Check sheet for the modelled part. Datum: model origin and axes. Units: mm. Round coordinates to 2 decimals unless told otherwise and drop trailing zeros. Order: outer loops, then holes, each group sorted by start corner. A loop starts at its lowest first (then second) coordinate and runs counter-clockwise, first axis right, second up.
```python
from build123d import *

# Parameters (mm, degrees)
F0_R     = 4.5
F0_R_2   = 30.25
F0_W     = 44
F0_H     = 3
F1_DEPTH = 4
F2_R     = 15
F3_R     = 1


with BuildPart() as f1:
    # F0 (on Top) → F1 (new body)
    with BuildSketch(Plane.XY):
        with BuildLine():
            ThreePointArc((-43.501786, 35.001786), (-35.001786, 26.501786), (-26.501786, 35.001786))
            ThreePointArc((-26.501786, 35.001786), (-28.991378, 41.012193), (-35.001786, 43.501786))
            ThreePointArc((-35.001786, 43.501786), (-39.901995, 41.94714), (-43.009713, 37.851891))
            ThreePointArc((-43.009713, 37.851891), (-43.377864, 36.447921), (-43.501786, 35.001786))
        make_face()
        with Locations((-35.001786, 35.001786)):
            Circle(F0_R, mode=Mode.SUBTRACT)
        with BuildLine():
            ThreePointArc((-35.001786, 43.501786), (-28.991378, 41.012193), (-26.501786, 35.001786))
            ThreePointArc((-26.501786, 35.001786), (-35.001786, 26.501786), (-43.501786, 35.001786))
            Line((-43.501786, 35.001786), (-43.501786, -35.001786))
            ThreePointArc((-43.501786, -35.001786), (-35.001786, -26.501786), (-26.501786, -35.001786))
            ThreePointArc((-26.501786, -35.001786), (-28.991378, -41.012193), (-35.001786, -43.501786))
            Line((-35.001786, -43.501786), (35.001786, -43.501786))
            ThreePointArc((35.001786, -43.501786), (28.991378, -28.991378), (43.501786, -35.001786))
            Line((43.501786, -35.001786), (43.501786, 35.001786))
            ThreePointArc((43.501786, 35.001786), (28.991378, 28.991378), (35.001786, 43.501786))
            Line((35.001786, 43.501786), (-35.001786, 43.501786))
        make_face()
        Circle(F0_R_2, mode=Mode.SUBTRACT)
        with BuildLine():
            Line((-43.501786, -35.001786), (-43.501786, 35.001786))
            ThreePointArc((-43.501786, 35.001786), (-43.377864, 36.447921), (-43.009713, 37.851891))
            Line((-43.009713, 37.851891), (-51.498214, 14.001786))
            Line((-51.498214, 14.001786), (-51.498214, -6.998214))
            Line((-51.498214, -6.998214), (-43.198922, -37.250552))
            ThreePointArc((-43.198922, -37.250552), (-43.42573, -36.13632), (-43.501786, -35.001786))
        make_face()
        with BuildLine():
            ThreePointArc((43.501786, 35.001786), (41.012193, 41.012193), (35.001786, 43.501786))
            ThreePointArc((35.001786, 43.501786), (28.991378, 28.991378), (43.501786, 35.001786))
        make_face()
        with Locations((35.001786, 35.001786)):
            Circle(F0_R, mode=Mode.SUBTRACT)
        with BuildLine():
            ThreePointArc((-26.501786, -35.001786), (-35.001786, -26.501786), (-43.501786, -35.001786))
            ThreePointArc((-43.501786, -35.001786), (-43.42573, -36.13632), (-43.198922, -37.250552))
            ThreePointArc((-43.198922, -37.250552), (-40.156176, -41.760651), (-35.001786, -43.501786))
            ThreePointArc((-35.001786, -43.501786), (-28.991378, -41.012193), (-26.501786, -35.001786))
        make_face()
        with Locations((-35.001786, -35.001786)):
            Circle(F0_R, mode=Mode.SUBTRACT)
        with BuildLine():
            ThreePointArc((35.001786, -43.501786), (41.012193, -41.012193), (43.501786, -35.001786))
            ThreePointArc((43.501786, -35.001786), (28.991378, -28.991378), (35.001786, -43.501786))
        make_face()
        with Locations((35.001786, -35.001786)):
            Circle(F0_R, mode=Mode.SUBTRACT)
        Polygon((35.001786, -43.501786), (-35.001786, -43.501786), (-35.001786, -45.501786), (-21.498214, -45.501786), (22.501786, -45.501786), (35.001786, -45.501786), align=None)
        with Locations((0.501786, -47.001786)):
            Rectangle(F0_W, F0_H)
    extrude(amount=F1_DEPTH)

    # F2
    f2_edges = [f1.edges().sort_by_distance(p)[0] for p in [
        (-51.498214, 14.001786, 2),
        (-51.498214, -6.998214, 2),
    ]]
    fillet(f2_edges, radius=F2_R)

    # F3
    f3_edges = [f1.edges().sort_by_distance(p)[0] for p in [
        (-35.001786, -43.501786, 2),
        (-21.498214, -45.501786, 2),
        (22.501786, -45.501786, 2),
        (35.001786, -43.501786, 2),
        (-35.001786, -45.501786, 2),
        (-21.498214, -48.501786, 2),
        (22.501786, -48.501786, 2),
        (35.001786, -45.501786, 2),
    ]]
    fillet(f3_edges, radius=F3_R)


solid = f1.part
```
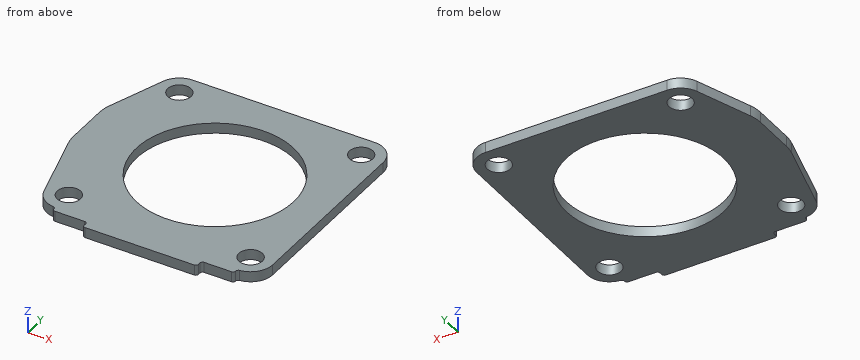
Item 1: Sectioned sample at B-B (x = 0). Record the cut outline in (y, z).
Answer:
outline: (-48.5, 0) - (-30.25, 0) - (-30.25, 4) - (-48.5, 4) - close; (30.25, 0) - (43.5, 0) - (43.5, 4) - (30.25, 4) - close
Item 2: Sectioned sample at A-A (y = 0). Record the cut outline in (x, z), and give its area (3 significant figures).
Answer:
outline: (-51.5, 0) - (-30.25, 0) - (-30.25, 4) - (-51.5, 4) - close; (30.25, 0) - (43.5, 0) - (43.5, 4) - (30.25, 4) - close
area: 138 mm2
Item 3: Sectioned sample at D-D (y = -32.5). Record the cut outline in (x, z), and give its area (3 significant figures).
Answer:
outline: (-44.5, 0) - (-38.74, 0) - (-38.74, 4) - (-44.5, 4) - close; (-31.26, 0) - (31.26, 0) - (31.26, 4) - (-31.26, 4) - close; (38.74, 0) - (43.5, 0) - (43.5, 4) - (38.74, 4) - close
area: 292 mm2
Item 4: Scan lines: line 1 along X through (y, z) = (-39, 1.35); line 2 along Y through (x, z) = (-34.5, 1.1); line 3 along Y through (x, z) = (20, 3.35). Record each from-to range of solid material in increasing order.
Answer:
line 1: x = -42.5 to -37.07, -32.94 to 32.94, 37.07 to 42.5
line 2: y = -45.37 to -39.47, -30.53 to 30.53, 39.47 to 43.5
line 3: y = -48.5 to -22.69, 22.69 to 43.5
Item 5: Sectioned sample at C-C (z = 1.8). State how many separate pieces and enclosed holes the cut face has, and give its area (3 significant figures).
Answer:
separate pieces: 1
enclosed holes: 5
area: 5,020 mm2
Item 6: Go/stop test with flat-tipped pins: P1, Ø8, axis at x = 35, y = -35, coming from the +Z side; P2, Ø0.5, axis at y = -47, z = 1.5, coming from the -X side; P3, Ø0.5, axis at y = -47, z = 1.5, coming from the +X side. Record where each tip stops, or that it passes through.
Answer:
P1: passes through
P2: stops at x = -21.5
P3: stops at x = 22.5
